For this review, take the finished solid that the model builds, in its own axes (mm). A direction names the side the tool comes from. Round coordinates to 2 decimals unless told otherwise and drop trailing zeros. Order: outer loops, then holes, each group sorted by start corner. A loop starts at its lowest first (then second) coordinate and runs counter-clockwise, first axis right, second up. Notation, with made-up numbers: (85, 70.25) - (112, 70.25) arc R26 cw to (112, 103.25) - close; hole circle Ø10 at (82.25, 25). An arc over 180 degrees is marked (long way). Write each question's results on one line, items separated by ' | '. Start each with the question number.
(1) For faces 5 (the flat face through (-3.131, 5.525, 10.846)), 6 (the cylindrical face through (4.42, 0.81, 14.95)), list the 3-axis set-ups (+Z, -Z, +X, -X, +Y, -Y) from which the entire face can be reached by the end or side of a thin tool; tool diameter is ignored.
(2) Take a section at A-A, the plane y = 0. Give the boundary of the cut face in (x, z), plus the area to 3 significant figures.
(3) For L1, parallel to Z at x = 4.9, y = 0; L2, parallel to Y at x = 4.85, z = 5.5; L3, parallel to Y at x = -2.25, z = 19.5, list the stretches that pass through material, from the lowest coordinate up. Write a range as from..to.
(4) Draft analysis for pull direction X (two halves, no side actions). For faces 1 (the cylindrical face through (4.42, -0.38, 3.79)), 2 (the cylindrical face through (-3, 0, 11)), 3 (the flat face through (-3.219, -5.474, 10.846)), 4 (the flat face through (6.35, 0, 11)), state which applies: pulls with the +X half, pulls with the -X half, needs draft (parallel to the pull), parting line crosses it, or undercut.
(5) Take a section at D-D, the plane y = -2. Give the boundary of the cut face in (x, z), plus the area to 3 significant figures.
(6) Insertion check: pin 1 Ø6 at (x, z) = (1, 16.5) entering from +Y; pin 2 Ø5 at (x, z) = (-1, 9.5) entering from -Y. Each pin has a flat end and moves straight along its axis. Give the tip position at first contact, or say it passes through.
(7) Take a section at C-C, the plane z = 5.5. Give the boundary of the cut face in (x, y), plus the area to 3 significant figures.
(8) Take a section at B-B, the plane x = -0.5. Give the boundary of the cut face in (y, z).
```python
from build123d import *

# Parameters (mm, degrees)
ESQUISSE1_R             = 3
BOSS_EXTRU_1_DEPTH      = 22
ESQUISSE3_R             = 1.75
ENL_V_MAT_EXTRU_1_DEPTH = 4.5


with BuildPart() as part:
    # Esquisse1 → Boss.-Extru.1 (new body)
    with BuildSketch(Plane.XY):
        Polygon((0, 7.332348419), (-6.35, 3.666174209), (-6.35, -3.666174209), (0, -7.332348419), (6.35, -3.666174209), (6.35, 3.666174209), align=None)
        Circle(ESQUISSE1_R, mode=Mode.SUBTRACT)
    extrude(amount=BOSS_EXTRU_1_DEPTH)

    # Esquisse3 → Enlèv. mat.-Extru.1 (cut)
    with BuildSketch(Plane(origin=(6.35, 0, 0), x_dir=(0, 0, -1), z_dir=(1, 0, 0))):
        with Locations(Location((-5.5, 0, 0), (0, 0, 90))):
            Circle(ESQUISSE3_R)
        with Locations(Location((-16.5, 0, 0), (0, 0, 90))):
            Circle(ESQUISSE3_R)
    extrude(amount=-ENL_V_MAT_EXTRU_1_DEPTH, mode=Mode.SUBTRACT)


solid = part.part
```
Results below:
1) face 5: +Z, -Z, -X, +Y | face 6: +X
2) outline: (-6.35, 0) - (-3, 0) - (-3, 22) - (-6.35, 22) - close; (3, 0) - (6.35, 0) - (6.35, 3.75) - (3, 3.75) - close; (3, 7.25) - (6.35, 7.25) - (6.35, 14.75) - (3, 14.75) - close; (3, 18.25) - (6.35, 18.25) - (6.35, 22) - (3, 22) - close | area: 124 mm^2
3) L1: z = 0..3.75, 7.25..14.75, 18.25..22 | L2: y = -4.53..-1.75, 1.75..4.53 | L3: y = -6.03..-1.98, 1.98..6.03
4) face 1: needs draft | face 2: undercut | face 3: pulls with the -X half | face 4: pulls with the +X half
5) outline: (-6.35, 0) - (-2.24, 0) - (-2.24, 22) - (-6.35, 22) - close; (2.24, 0) - (6.35, 0) - (6.35, 22) - (2.24, 22) - close | area: 181 mm^2
6) pin 1: stops at y = 7.33 | pin 2: stops at y = -7.33
7) outline: (-6.35, -3.67) - (0, -7.33) - (6.35, -3.67) - (6.35, -1.75) - (2.44, -1.75) arc R3 cw (long way) to (2.44, 1.75) - (6.35, 1.75) - (6.35, 3.67) - (0, 7.33) - (-6.35, 3.67) - close | area: 99.1 mm^2
8) outline: (-7.04, 0) - (-2.96, 0) - (-2.96, 22) - (-7.04, 22) - close; (2.96, 0) - (7.04, 0) - (7.04, 22) - (2.96, 22) - close
